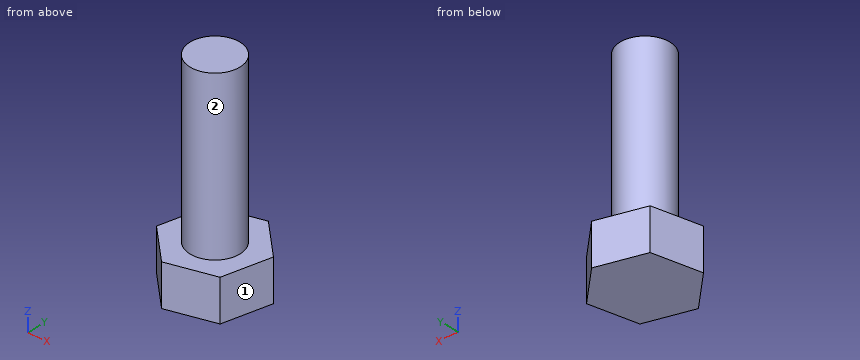
from build123d import *

# Parameters (mm, degrees)
F0_R     = 3
F1_DEPTH = 20
F2_R     = 3
F3_DEPTH = 5


with BuildPart() as f1:
    # F0 (on Top) → F1 (new body)
    with BuildSketch(Plane.XY):
        Circle(F0_R)
    extrude(amount=F1_DEPTH)

    # F2 (on face) → F3 (join)
    with BuildSketch(Plane(origin=(0, 0, 0), x_dir=(1, 0, 0), z_dir=(0, 0, -1))):
        Polygon((1.3301522364, -5.6181872843), (5.5305690296, -1.6571480145), (4.2004167932, 3.9610392698), (-1.3301522364, 5.6181872843), (-5.5305690296, 1.6571480145), (-4.2004167932, -3.9610392698), align=None)
        Circle(F2_R, mode=Mode.SUBTRACT)
        Circle(F2_R)
    extrude(amount=F3_DEPTH)


solid = f1.part
Verification items for the finished model (mm, model axes). Face numbers are marked on the shaded views. A direction names the side the tool comes from. Round coordinates to 2 decimals unless told otherwise and drop trailing zeros. Loops run counter-clockwise (first coordinate to the right, second up) from the corner with the lowest first, then second, coordinate; pieces in that order, holes last. Notation, with made-up numbers: M 82.5,28 L 106.5,28 A27 cw 106.5,57 Z; hole C -23,25.25 d5. An arc over 180 degrees is marked long. Write each question's results on one line, items separated by ' | '.
1) Scan lines: L1, parallel to Y at x = 2.5, z = 13; L2, parallel to Z at x = -3.5, y = 3.5. Record each from-to range of solid material in increasing order. Write a range as from..to.
Checks:
L1: y = -1.66..1.66 | L2: z = -5..0
2) Section check C-C on x = 0. Record the boundary of the cut face in (y, z), then the cut area to 3 significant figures.
Checks:
outline: M -5.22,-5 L 5.22,-5 L 5.22,0 L 3,0 L 3,20 L -3,20 L -3,0 L -5.22,0 Z | area: 172 mm2
3) Section check D-D on z = 7.75. Record the boundary of the cut face in (x, y), then the cut area to 3 significant figures.
Checks:
outline: C 0,0 d6 | area: 28.3 mm2
4) Section check B-B on z = -1.5. Record the boundary of the cut face in (x, y), then the cut area to 3 significant figures.
Checks:
outline: M -5.53,-1.66 L -1.33,-5.62 L 4.2,-3.96 L 5.53,1.66 L 1.33,5.62 L -4.2,3.96 Z | area: 86.6 mm2
5) Access from +Z, -Z, +X, -X, +Y, -Y to the whole of each face (thin tool, end or side, straight path). Record for the marked faces 1 and 2.
Checks:
face 1: +Z, -Z, +X, -Y | face 2: +Z
6) Gauge pin test, flat ends, axial feed: P1, Ø5, axis at y = -2.5, z = 15.5, coming from the -X side; P2, Ø2, axis at y = -1, z = 7.5, coming from the +X side; P3, Ø2, axis at x = -1, z = 8, coming from the -Y side. Record the tip position at first contact, or that the pin passes through.
Checks:
P1: stops at x = -3 | P2: stops at x = 3 | P3: stops at y = -3
7) Section check A-A on y = 2.25. Record the boundary of the cut face in (x, z).
Checks:
outline: M -4.61,-5 L 4.9,-5 L 4.9,0 L 1.98,0 L 1.98,20 L -1.98,20 L -1.98,0 L -4.61,0 Z
